Model file for the job. Use its own axes, mm. Face numbers are marked on the shaded views. A direction names the side the tool comes from. Coordinates: 2 decimals unless noted, no trailing zeros. Order: outer loops, then holes, each group sorted by start corner. A loop starts at its lowest first (then second) coordinate and runs counter-clockwise, first axis right, second up. Notation, with made-up numbers: (29, 22.25) -> (54, 22.25) arc R14 cw to (54, 41.25) -> close; hole circle Ø8 at (-11, 58). An arc over 180 degrees is marked (long way). Write item = value, one per line. Start each with the question number.
Q1. Cut at D-D, the plane z = -175. List the corners of the cut face in (x, y), plus the area to 3 significant figures.
Q2. Cut at B-B, the plane z = -34. List the corners of the cut face in (x, y), plus the area to 3 significant figures.
Q3. Cut at C-C, the plane y = 67. Give the number of separate pieces and of enclosed holes in the cut face, plus the area to 3 significant figures.
Q4. Mould opens along X. For the marked faces 1, 2 and 3 say: +X half, -X half, draft (parallel to the pull), parting line (faces both ways), or undercut.
Q5. Flat gauge pins, fed straight in: pin 1 (3 mm diameter, centred on x = 58.5, z = -101.5, fed in from -Y); pin 2 (18 mm diameter, centred on y = 15, z = -107.5, fed in from -X); pin 3 (2 mm diameter, centred on x = 21.5, z = -172.5, fed in from -Y). Where does each tip first touch, or does it go through?
Q6. 3-axis set-ups, long thin cutter, end or side, ignore diameter. For the marked faces 4 and 5: which of +Z, -Z, +X, -X, +Y, -Y reach the whole face in a straight line?
Q7. Wall check: line 1 (Z direction, x = 65, y = 30); line 2 (X direction, y = 47.5, z = -167.5); line 3 (Z direction, x = 51, y = 58.5). Give the ranges that are in metal, low to high. Write a range as from..to.
Autodesk Inventor part; units mm, degrees
ref_plane "YZ Plane" through (0, 0, 0) normal (1, 0, 0) x (0, 1, 0)
ref_plane "XZ Plane" through (0, 0, 0) normal (0, 1, 0) x (-1, 0, 0)
ref_plane "XY Plane" through (0, 0, 0) normal (0, 0, 1) x (1, 0, 0)
sketch "Sketch1" plane through (0, 0, 0) normal (0, 1, 0) x (-1, 0, 0)
  line L0 (0, 0) -> (-80, 0)
  line L1 (-80, 0) -> (-80, -202)
  line L2 (-80, -202) -> (0, -202)
  line L3 (0, -202) -> (0, 0)
  line L4 (-4, -4) -> (-38, -4)
  line L5 (-38, -4) -> (-38, -39.6)
  line L6 (-38, -39.6) -> (-4, -39.6)
  line L7 (-4, -39.6) -> (-4, -4)
  line L8 (-4, -43.6) -> (-38, -43.6)
  line L9 (-38, -43.6) -> (-38, -79.2)
  line L10 (-38, -79.2) -> (-4, -79.2)
  line L11 (-4, -79.2) -> (-4, -43.6)
  line L12 (-4, -83.2) -> (-38, -83.2)
  line L13 (-38, -83.2) -> (-38, -118.8)
  line L14 (-38, -118.8) -> (-4, -118.8)
  line L15 (-4, -118.8) -> (-4, -83.2)
  line L16 (-4, -122.8) -> (-38, -122.8)
  line L17 (-38, -122.8) -> (-38, -158.4)
  line L18 (-38, -158.4) -> (-4, -158.4)
  line L19 (-4, -158.4) -> (-4, -122.8)
  line L20 (-4, -162.4) -> (-38, -162.4)
  line L21 (-38, -162.4) -> (-38, -198)
  line L22 (-38, -198) -> (-4, -198)
  line L23 (-4, -198) -> (-4, -162.4)
  line L24 (-76, -198) -> (-42, -198)
  line L25 (-42, -162.4) -> (-76, -162.4)
  line L26 (-42, -198) -> (-42, -162.4)
  line L27 (-76, -162.4) -> (-76, -198)
  line L28 (-76, -158.4) -> (-42, -158.4)
  line L29 (-76, -122.8) -> (-76, -158.4)
  line L30 (-42, -122.8) -> (-76, -122.8)
  line L31 (-42, -158.4) -> (-42, -122.8)
  line L32 (-76, -118.8) -> (-42, -118.8)
  line L33 (-76, -83.2) -> (-76, -118.8)
  line L34 (-42, -118.8) -> (-42, -83.2)
  line L35 (-42, -4) -> (-76, -4)
  line L36 (-76, -4) -> (-76, -39.6)
  line L37 (-76, -39.6) -> (-42, -39.6)
  line L38 (-42, -83.2) -> (-76, -83.2)
  line L39 (-76, -79.2) -> (-42, -79.2)
  line L40 (-42, -43.6) -> (-76, -43.6)
  line L41 (-76, -43.6) -> (-76, -79.2)
  line L42 (-42, -79.2) -> (-42, -43.6)
  line L43 (-42, -39.6) -> (-42, -4)
  dimension "d0" = 34
  dimension "d1" = 35.6
  dimension "d2" = 4
  dimension "d3" = 4
  dimension "d6" = 39.6
  dimension "d11" = 4
  dimension "d14" = 38
  dimension "d19" = 4
extrude "Extrusion1" add sketch "Sketch1" along normal blind 70
sketch "Sketch2" plane through (0, 70, 0) normal (0, 1, 0) x (1, 0, 0)
  line L0 (0, 0) -> (80, 0)
  line L1 (0, 202) -> (0, 0)
  line L2 (80, 0) -> (80, 202)
  line L3 (80, 202) -> (0, 202)
extrude "Extrusion2" add sketch "Sketch2" along normal blind 4
ref_plane "Work Plane4" through (40, 0, -202) normal (-1, 0, 0) x (0, 0, 1)
fillet "Fillet1" radius 15 40 edges at (21, 70, -198) (4, 70, -180.2) (59, 70, -198) (42, 70, -180.2) (59, 70, -158.4) (42, 70, -140.6) (21, 70, -158.4) (4, 70, -140.6) (59, 70, -118.8) (42, 70, -101) (21, 70, -118.8) (4, 70, -101) (21, 70, -79.2) (4, 70, -61.4) (59, 70, -79.2) (42, 70, -61.4) (59, 70, -39.6) (42, 70, -21.8) (21, 70, -39.6) (4, 70, -21.8) (76, 70, -21.8) (59, 70, -4) (38, 70, -21.8) (21, 70, -4) (38, 70, -61.4) (21, 70, -43.6) (76, 70, -61.4) (59, 70, -43.6) (76, 70, -101) (59, 70, -83.2) (76, 70, -140.6) (59, 70, -122.8) (38, 70, -140.6) (21, 70, -122.8) (38, 70, -180.2) (21, 70, -162.4) (76, 70, -180.2) (59, 70, -162.4) (38, 70, -101) (21, 70, -83.2)
properties part number "Contenedor B" material "ABS Plastic"
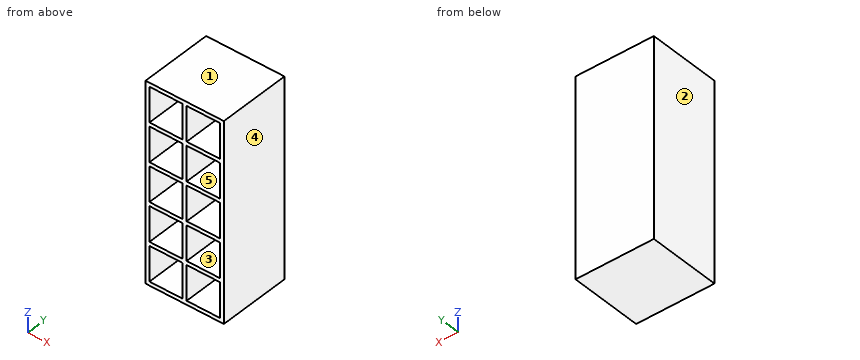
Here are the results:
q1.outline = (0, 0) -> (4, 0) -> (4, 55) arc R15 cw to (16.6, 69.81) -> (25.4, 69.81) arc R15 cw to (38, 55) -> (38, 0) -> (42, 0) -> (42, 55) arc R15 cw to (54.6, 69.81) -> (63.4, 69.81) arc R15 cw to (76, 55) -> (76, 0) -> (80, 0) -> (80, 74) -> (0, 74) -> close
q1.area = 1,360 mm²
q2.outline = (0, 0) -> (4, 0) -> (4, 55) arc R15 cw to (9.6, 66.69) -> (32.4, 66.69) arc R15 cw to (38, 55) -> (38, 0) -> (42, 0) -> (42, 55) arc R15 cw to (47.6, 66.69) -> (70.4, 66.69) arc R15 cw to (76, 55) -> (76, 0) -> (80, 0) -> (80, 74) -> (0, 74) -> close
q2.area = 1,460 mm²
q3.separate_pieces = 1
q3.enclosed_holes = 10
q3.area = 11,000 mm²
q4.face_1 = draft
q4.face_2 = -X half
q4.face_3 = undercut
q5.pin_1 = 70
q5.pin_2 = 0
q5.pin_3 = 68.79
q6.face_4 = +Z, -Z, +X, +Y, -Y
q6.face_5 = -Y
q7.line_1 = -202..-198, -162.4..-158.4, -122.8..-118.8, -83.2..-79.2, -43.6..-39.6, -4..0
q7.line_2 = 0..4, 38..42, 76..80
q7.line_3 = -202..-197.59, -162.81..-157.99, -123.21..-118.39, -83.61..-78.79, -44.01..-39.19, -4.41..0
